CAD build for the part. Positions are in the model's coordinates, mm. Round coordinates to 2 decimals unless told otherwise and drop trailing zeros. Put each result on its own line as item: value. Start each with the question number.
from build123d import *

# Parameters (mm, degrees)
BOSS_EXTRUDE1_DEPTH = 3.175
SKETCH2_R           = 2.5527
CUT_EXTRUDE1_DEPTH  = 4.175
CUT_EXTRUDE2_DEPTH  = 4.175
SKETCH4_R           = 2.5527
CUT_EXTRUDE3_DEPTH  = 4.175


with BuildPart() as part:
    # Sketch1 → Boss-Extrude1 (new body)
    with BuildSketch(Plane.XY):
        with BuildLine():
            Line((-152.4, 136.525), (-128.098009656, 162.977004026))
            Line((-128.098009656, 162.977004026), (120.423210344, 162.977004026))
            ThreePointArc((120.423210344, 162.977004026), (124.628339443, 147.208762232), (140.874895001, 145.669284239))
            Line((140.874895001, 145.669284239), (152.4, 136.525))
            Line((152.4, 136.525), (152.4, 39.6875))
            Line((152.4, 39.6875), (101.6, 39.6875))
            Line((101.6, 39.6875), (101.6, -39.6875))
            Line((101.6, -39.6875), (152.4, -39.6875))
            Line((152.4, -39.6875), (152.4, -136.525))
            Line((152.4, -136.525), (140.874895001, -145.669284239))
            ThreePointArc((140.874895001, -145.669284239), (124.628339443, -147.208762232), (120.423210344, -162.977004026))
            Line((120.423210344, -162.977004026), (-128.098009656, -162.977004026))
            Line((-128.098009656, -162.977004026), (-152.4, -136.525))
            Line((-152.4, -136.525), (-152.4, 136.525))
        make_face()
    extrude(amount=BOSS_EXTRUDE1_DEPTH)

    # Sketch2 → Cut-Extrude1 (cut, through all)
    with BuildSketch(Plane.XY.offset(3.175)):
        with Locations((-102.698009656, 152.829704026)):
            Circle(SKETCH2_R)
        with Locations((-77.298009656, 152.829704026)):
            Circle(SKETCH2_R)
        with Locations((-51.898009656, 152.829704026)):
            Circle(SKETCH2_R)
        with Locations((-26.498009656, 152.829704026)):
            Circle(SKETCH2_R)
        with Locations((-1.098009656, 152.829704026)):
            Circle(SKETCH2_R)
        with Locations((24.301990344, 152.829704026)):
            Circle(SKETCH2_R)
        with Locations((49.701990344, 152.829704026)):
            Circle(SKETCH2_R)
        with Locations((75.101990344, 152.829704026)):
            Circle(SKETCH2_R)
        with Locations((-51.898009656, -152.829704026)):
            Circle(SKETCH2_R)
        with Locations((-77.298009656, -152.829704026)):
            Circle(SKETCH2_R)
        with Locations((-102.698009656, -152.829704026)):
            Circle(SKETCH2_R)
        with Locations((-26.498009656, -152.829704026)):
            Circle(SKETCH2_R)
        with Locations((-1.098009656, -152.829704026)):
            Circle(SKETCH2_R)
        with Locations((24.301990344, -152.829704026)):
            Circle(SKETCH2_R)
        with Locations((49.701990344, -152.829704026)):
            Circle(SKETCH2_R)
        with Locations((75.101990344, -152.829704026)):
            Circle(SKETCH2_R)
    extrude(amount=-CUT_EXTRUDE1_DEPTH, mode=Mode.SUBTRACT)

    # Sketch3 → Cut-Extrude2 (cut, through all)
    with BuildSketch(Plane.XY.offset(3.175)):
        Polygon((-133.286983573, 124.204793052), (-139.572032875, 127.981231667), (-145.985049302, 124.426438614), (-146.113016427, 117.095206948), (-139.827967125, 113.318768333), (-133.414950698, 116.873561386), align=None)
    extrude(amount=-CUT_EXTRUDE2_DEPTH, mode=Mode.SUBTRACT)

    # Sketch4 → Cut-Extrude3 (cut, through all)
    with BuildSketch(Plane(origin=(0, 0, 0), x_dir=(-1, 0, 0), z_dir=(0, 0, -1))):
        with Locations((139.7, 76.2)):
            Circle(SKETCH4_R)
        with Locations((139.7, 50.8)):
            Circle(SKETCH4_R)
        with Locations((139.7, 25.4)):
            Circle(SKETCH4_R)
        with Locations((139.7, 0)):
            Circle(SKETCH4_R)
        with Locations((139.7, -25.4)):
            Circle(SKETCH4_R)
        with Locations((139.7, -50.8)):
            Circle(SKETCH4_R)
        with Locations((139.7, -76.2)):
            Circle(SKETCH4_R)
    extrude(amount=-CUT_EXTRUDE3_DEPTH, mode=Mode.SUBTRACT)


solid = part.part
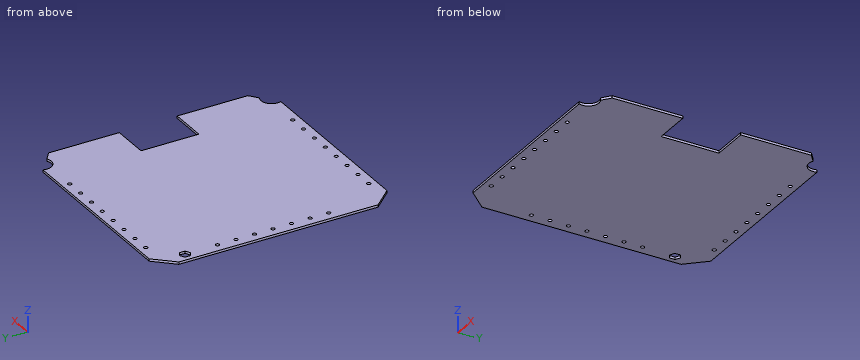
(1) Drill centre lines: line 1 along Y through (x, z) = (116, 1.6); line 2 along Y through (x, z) = (133, 1.9); line 3 along X through (y, z) = (120.5, 0.35). Where is each one in solid material? Low to high.
(2) Cut at A-A on z = 2.6. Count the separate pieces of the cut face and the enclosed holes in it, and give its area (3 significant figures).
(3) Flat gauge pins, fed straight in: pin 1 Ø1 at (x, z) = (120.5, 2.5) entering from -Y; pin 2 Ø4 at (x, y) = (24.3, -152.83) entering from +Z. Where does each tip first touch, or does it go through?
Taken from the geometry:
1. line 1: -162.98 to -39.69, 39.69 to 162.98
1. line 2: -143.85 to -39.69, 39.69 to 143.85
1. line 3: -152.4 to -146.05, -133.35 to 152.4
2. separate pieces: 1
2. enclosed holes: 24
2. area: 92,800 mm2
3. pin 1: y = -162.98
3. pin 2: through
